Source: CAD feature listing. Evaluate the final solid. Frame: model axes, mm. Round coordinates to 2 decimals unless told otherwise and drop trailing zeros. Order: outer loops, then holes, each group sorted by start corner. A loop starts at its lowest first (then second) coordinate and runs counter-clockwise, first axis right, second up. Notation, with made-up numbers: M -36.5,-9.5 L 9.5,-9.5 A21 ccw 9.5,3.5 Z; hole C 18,-29.75 d3. An arc over 180 degrees is marked long. Answer as CSV lines item,"result". Start each with the question number.
Item 1: Section query C-C on x = 4.5. Return the cut outline in (y, z).
Item 2: Section query B-B on x = 9. Return the cut outline in (y, z).
Item 3: Section query A-A on y = 0.4. Return the cut outline in (x, z).
Item 4: Line query: line 1 (X direction, y = 0.4, z = 5.5); line 2 (X direction, y = 0.35, z = 6) (3 decimals); line 3 (Y direction, x = 11.5, z = 4). Output: solid intervals per line, ascending. Write a range as [from, to].
Autodesk Inventor part; units mm, degrees
ref_plane "YZ Plane" through (0, 0, 0) normal (1, 0, 0) x (0, 1, 0)
ref_plane "XZ Plane" through (0, 0, 0) normal (0, 1, 0) x (-1, 0, 0)
ref_plane "XY Plane" through (0, 0, 0) normal (0, 0, 1) x (1, 0, 0)
sketch "Sketch1" plane through (0, 0, 0) normal (0, 0, 1) x (1, 0, 0)
  line L0 (10, 0) -> (10.1908, 0)
  line L1 (10.359, 0.0918) -> (10.691, 0.6082)
  line L2 (11.809, 0.6082) -> (12.141, 0.0918)
  line L3 (10.8592, 0.7) -> (11.6408, 0.7)
  arc A0 (11.809, 0.6082) -> (11.6408, 0.7) centre (11.6408, 0.5) ccw
  arc A1 (10.8592, 0.7) -> (10.691, 0.6082) centre (10.8592, 0.5) ccw
  line L4 (12.3092, 0) -> (12.5, 0)
  arc A2 (10.1908, 0) -> (10.359, 0.0918) centre (10.1908, 0.2) ccw
  arc A3 (12.141, 0.0918) -> (12.3092, 0) centre (12.3092, 0.2) ccw
  line L5 (7.5, 0) -> (7.6908, 0)
  line L6 (7.859, 0.0918) -> (8.191, 0.6082)
  line L7 (9.309, 0.6082) -> (9.641, 0.0918)
  line L8 (8.3592, 0.7) -> (9.1408, 0.7)
  arc A4 (9.309, 0.6082) -> (9.1408, 0.7) centre (9.1408, 0.5) ccw
  arc A5 (8.3592, 0.7) -> (8.191, 0.6082) centre (8.3592, 0.5) ccw
  line L9 (9.8092, 0) -> (10, 0)
  arc A6 (7.6908, 0) -> (7.859, 0.0918) centre (7.6908, 0.2) ccw
  arc A7 (9.641, 0.0918) -> (9.8092, 0) centre (9.8092, 0.2) ccw
  line L10 (5, 0) -> (5.1908, 0)
  line L11 (5.359, 0.0918) -> (5.691, 0.6082)
  line L12 (6.809, 0.6082) -> (7.141, 0.0918)
  line L13 (5.8592, 0.7) -> (6.6408, 0.7)
  arc A8 (6.809, 0.6082) -> (6.6408, 0.7) centre (6.6408, 0.5) ccw
  arc A9 (5.8592, 0.7) -> (5.691, 0.6082) centre (5.8592, 0.5) ccw
  line L14 (7.3092, 0) -> (7.5, 0)
  arc A10 (5.1908, 0) -> (5.359, 0.0918) centre (5.1908, 0.2) ccw
  arc A11 (7.141, 0.0918) -> (7.3092, 0) centre (7.3092, 0.2) ccw
  line L15 (2.5, 0) -> (2.6908, 0)
  line L16 (2.859, 0.0918) -> (3.191, 0.6082)
  line L17 (4.309, 0.6082) -> (4.641, 0.0918)
  line L18 (3.3592, 0.7) -> (4.1408, 0.7)
  arc A12 (4.309, 0.6082) -> (4.1408, 0.7) centre (4.1408, 0.5) ccw
  arc A13 (3.3592, 0.7) -> (3.191, 0.6082) centre (3.3592, 0.5) ccw
  line L19 (4.8092, 0) -> (5, 0)
  arc A14 (2.6908, 0) -> (2.859, 0.0918) centre (2.6908, 0.2) ccw
  arc A15 (4.641, 0.0918) -> (4.8092, 0) centre (4.8092, 0.2) ccw
  line L20 (0, 0) -> (0.1908, 0)
  line L21 (0.359, 0.0918) -> (0.691, 0.6082)
  line L22 (1.809, 0.6082) -> (2.141, 0.0918)
  line L23 (0.8592, 0.7) -> (1.6408, 0.7)
  arc A16 (1.809, 0.6082) -> (1.6408, 0.7) centre (1.6408, 0.5) ccw
  arc A17 (0.8592, 0.7) -> (0.691, 0.6082) centre (0.8592, 0.5) ccw
  line L24 (2.3092, 0) -> (2.5, 0)
  arc A18 (0.1908, 0) -> (0.359, 0.0918) centre (0.1908, 0.2) ccw
  arc A19 (2.141, 0.0918) -> (2.3092, 0) centre (2.3092, 0.2) ccw
  line L25 (12.5, 0) -> (12.5, 1.3)
  line L26 (12.5, 1.3) -> (0, 1.3)
  line L27 (0, 1.3) -> (0, 0)
  line L28 (7.3092, 0) -> (7.6908, 0)
  line L29 (9.8092, 0) -> (10.1908, 0)
  line L30 (12.3092, 0) -> (12.5, 0)
  line L31 (4.8092, 0) -> (5.1908, 0)
  line L32 (0, 0) -> (0.1908, 0)
  line L33 (2.3092, 0) -> (2.6908, 0)
  point P0 (0, 0)
  point P1 (10.3, 0)
  point P2 (12.2, 0)
  point P3 (7.8, 0)
  point P4 (9.7, 0)
  point P5 (5.3, 0)
  point P6 (7.2, 0)
  point P7 (2.8, 0)
  point P8 (4.7, 0)
  point P9 (0.3, 0)
  point P10 (2.2, 0)
  dimension "d14" = 10
  dimension "d5" = 0.3
  dimension "d7" = 0.2
  dimension "d8" = 0.2
  dimension "d11" = 2.5
  dimension "d16" = 1.3
extrude "Extrusion1" add sketch "Sketch1" along normal blind 10
pattern_of_one "Rectangular Pattern1"
properties part number "T2.5 belt-01" material "Rubber"
Results:
1,outline,"M 0.31,0 L 1.3,0 L 1.3,10 L 0.31,10 Z"
2,outline,"M 0.7,0 L 1.3,0 L 1.3,10 L 0.7,10 Z"
3,outline,"M 0,0 L 0.56,0 L 0.56,10 L 0,10 Z; M 1.94,0 L 3.06,0 L 3.06,10 L 1.94,10 Z; M 4.44,0 L 5.56,0 L 5.56,10 L 4.44,10 Z; M 6.94,0 L 8.06,0 L 8.06,10 L 6.94,10 Z; M 9.44,0 L 10.56,0 L 10.56,10 L 9.44,10 Z; M 11.94,0 L 12.5,0 L 12.5,10 L 11.94,10 Z"
4,line 1,"[0, 0.56], [1.94, 3.06], [4.44, 5.56], [6.94, 8.06], [9.44, 10.56], [11.94, 12.5]"
4,line 2,"[0, 0.525], [1.975, 3.025], [4.475, 5.525], [6.975, 8.025], [9.475, 10.525], [11.975, 12.5]"
4,line 3,"[0.7, 1.3]"
